The model under review builds one solid part; all positions refer to its coordinate system, in mm. Face numbers are marked on the shaded views. A direction names the side the tool comes from. Round coordinates to 2 decimals unless told otherwise and drop trailing zeros. Order: outer loops, then holes, each group sorted by start corner. A loop starts at its lowest first (then second) coordinate and runs counter-clockwise, first axis right, second up. Notation, with made-up numbers: (11, 0.25) -> (65, 0.25) arc R9 ccw to (65, 15.25) -> close; hole circle Ø8 at (-2.75, 13). An arc over 180 degrees is marked (long way). Use a Markdown table: item, result. Add a question column.
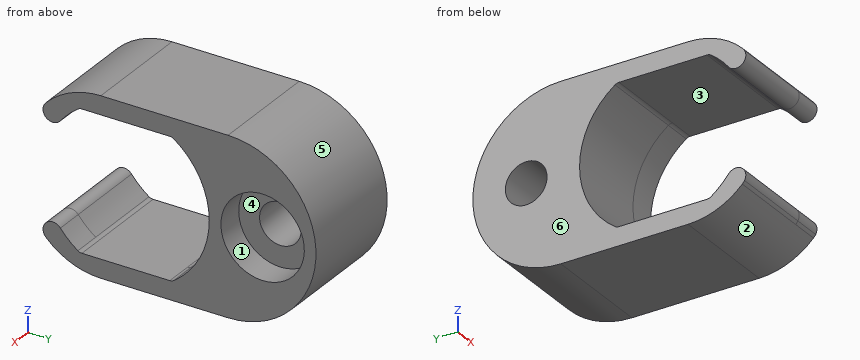
Autodesk Inventor part; units mm, degrees
ref_plane "Work Plane1" through (124.425, 27.025, -10.85) normal (1, 0, 0) x (0, 1, 0)
ref_plane "YZ Plane" through (0, 0, 0) normal (1, 0, 0) x (0, 1, 0)
ref_plane "XZ Plane" through (0, 0, 0) normal (0, 1, 0) x (-1, 0, 0)
sketch "Sketch1" plane through (0, 0, 0) normal (1, 0, 0) x (0, 1, 0)
  line L0 (14.875, -0.7) -> (14.875, 0.8967)
  line L1 (27.025, -0.7) -> (14.875, -0.7)
  line L2 (27.025, -10.85) -> (27.025, -0.7)
  line L3 (15.75, -10.85) -> (27.025, -10.85)
  line L4 (34.625, -12.1) -> (15.75, -12.1)
  line L5 (34.625, -3.2) -> (34.625, -12.1)
  line L6 (15.7197, 0.55) -> (30.875, 0.55)
  arc A0 (17.7877, -0.775) -> (17.5002, -0.8659) centre (17.7877, -1.275) ccw
  arc A1 (17.5002, -0.8659) -> (17.5002, -10.6841) centre (20.95, -5.775) ccw
  arc A2 (17.5002, -10.6841) -> (17.7877, -10.775) centre (17.7877, -10.275) ccw
  line L7 (17.7877, -10.775) -> (24.1123, -10.775)
  arc A3 (24.1123, -10.775) -> (24.3998, -10.6841) centre (24.1123, -10.275) ccw
  arc A4 (24.3998, -10.6841) -> (24.3998, -0.8659) centre (20.95, -5.775) ccw
  arc A5 (24.3998, -0.8659) -> (24.1123, -0.775) centre (24.1123, -1.275) ccw
  line L8 (24.1123, -0.775) -> (17.7877, -0.775)
  line L9 (26.95, -5.775) -> (26.95, -9.775)
  arc A6 (24.3998, -10.6841) -> (26.95, -5.775) centre (20.95, -5.775) ccw
  arc A7 (24.1123, -10.775) -> (24.3998, -10.6841) centre (24.1123, -10.275) ccw
  line L10 (25.95, -10.775) -> (24.1123, -10.775)
  arc A8 (25.95, -10.775) -> (26.95, -9.775) centre (25.95, -9.775) ccw
  line L11 (24.1123, -0.775) -> (25.95, -0.775)
  arc A9 (24.3998, -0.8659) -> (24.1123, -0.775) centre (24.1123, -1.275) ccw
  arc A10 (26.95, -5.775) -> (24.3998, -0.8659) centre (20.95, -5.775) ccw
  line L12 (26.95, -1.775) -> (26.95, -5.775)
  arc A11 (26.95, -1.775) -> (25.95, -0.775) centre (25.95, -1.775) ccw
  line L13 (14.95, -5.775) -> (14.95, -1.775)
  arc A12 (17.5002, -0.8659) -> (14.95, -5.775) centre (20.95, -5.775) ccw
  arc A13 (17.7877, -0.775) -> (17.5002, -0.8659) centre (17.7877, -1.275) ccw
  line L14 (15.95, -0.775) -> (17.7877, -0.775)
  arc A14 (15.95, -0.775) -> (14.95, -1.775) centre (15.95, -1.775) ccw
  line L15 (17.7877, -10.775) -> (15.95, -10.775)
  arc A15 (17.5002, -10.6841) -> (17.7877, -10.775) centre (17.7877, -10.275) ccw
  arc A16 (14.95, -5.775) -> (17.5002, -10.6841) centre (20.95, -5.775) ccw
  line L16 (14.95, -9.775) -> (14.95, -5.775)
  arc A17 (14.95, -9.775) -> (15.95, -10.775) centre (15.95, -9.775) ccw
  line L17 (26.95, -10.85) -> (14.95, -10.85)
  line L18 (14.95, -10.85) -> (14.95, -12.1)
  line L19 (14.95, -12.1) -> (26.95, -12.1)
  line L20 (26.95, -12.1) -> (26.95, -10.85)
  line L21 (20.95, -5.775) -> (14.95, -5.775)
  arc A18 (15.2429, -10.4821) -> (19.1488, -12.1) centre (19.1488, -6.5762) ccw
  arc A19 (15.8269, -8.8981) -> (14.95, -9.775) centre (15.8269, -9.775) ccw
  line L22 (14.95, -9.775) -> (15.8269, -8.8981) construction
  line L23 (14.95, -9.775) -> (16.1901, -9.775) construction
  line L24 (26.95, -0.7) -> (14.95, -0.7)
  line L25 (14.95, -0.7) -> (14.95, 0.55)
  line L26 (14.95, 0.55) -> (26.95, 0.55)
  line L27 (26.95, 0.55) -> (26.95, -0.7)
  arc A20 (19.1488, 0.55) -> (15.2429, -1.0679) centre (19.1488, -4.9738) ccw
  arc A21 (14.95, -1.775) -> (15.8269, -2.6519) centre (15.8269, -1.775) ccw
  line L28 (26.95, -12.1) -> (26.95, 0.55)
  line L29 (26.95, 0.55) -> (34.625, 0.55)
  line L30 (34.625, 0.55) -> (34.625, -12.1)
  line L31 (34.625, -12.1) -> (26.95, -12.1)
  line L32 (26.95, -5.775) -> (34.625, -5.775)
  circle A22 centre (30.7875, -5.775) radius 1.5
  circle A23 centre (30.7875, -5.775) radius 3
  arc A24 (28.3, -12.1) -> (34.625, -5.775) centre (28.3, -5.775) ccw
  arc A25 (34.625, -5.775) -> (28.3, 0.55) centre (28.3, -5.775) ccw
  line L33 (15.75, -12.1) -> (15.75, -10.85)
  arc A26 (34.625, -3.2) -> (30.875, 0.55) centre (30.875, -3.2) ccw
  arc A27 (14.8505, 1.3251) -> (15.7197, 0.55) centre (15.7197, 1.425) ccw
  arc A28 (14.875, 0.8967) -> (14.8505, 1.3251) centre (11.125, 0.8967) ccw
  circle A29 centre (30.7875, -5.775) radius 1.4375
  point P0 (0, 0)
  point P1 (15.8269, -8.8981)
  point P2 (19.1488, -12.1)
  point P3 (28.3, -12.1)
  point P4 (28.3, 0.55)
  point P5 (19.1488, 0.55)
  point P6 (15.2429, -1.0679)
  point P7 (15.8269, -2.6519)
  point P8 (15.75, -10.9306)
  point P9 (27.025, -5.775)
  point P10 (15.6492, -0.7)
  dimension "d0" = 1.25
  dimension "d1" = 45
  dimension "d2" = 3
  dimension "d3" = 6
ref_plane "Work Plane1" through (124.425, 27.025, -10.85) normal (1, 0, 0) x (0, 1, 0)
extrude "Extrusion1" add sketch "Sketch1" along normal blind 6 from surface at 124.425 contours A20 L6 L27 L1 | L1 L28 A11 L11 L8 L14 A14 A20 | L27 L6 A25 L32 A23 L2 L1 | L1 L2 L32 L12 L28 | A14 L14 A0 A1 A21 | L12 A4 A5 L11 A11 | L32 A23 A24 L4 L20 L3 L2 | L2 L3 L28 L9 L32 | L9 A8 L10 A3 A4 | A23 L32 A22 | L32 A22 A23 | L28 L3 L17 A18 A17 L15 L7 L10 A8 | A1 A2 L15 A17 A19 | L20 L4 A18 L33 L3 | L33 A18 L17
fillet "Fillet1" radius 0.7 2 edges at (127.425, 15.8269, -2.6519) (127.425, 15.8269, -8.8981)
sketch "Sketch2" plane through (130.425, 19.1488, -12.1) normal (1, 0, 0) x (0, 0, -1)
  arc A0 (-2.6078, -2.9087) -> (-1.8221, -4.0632) centre (-2.1741, -3.4581) ccw
  line L0 (0, 9.1512) -> (0, 0)
  line L1 (-12.65, 0) -> (-12.65, 9.1512)
  arc A1 (-11.0321, -3.9059) -> (-10.8279, -4.0632) centre (-10.325, -3.1988) ccw
  arc A2 (-11.2341, -1.6486) -> (-10.0422, -2.9087) centre (-6.325, 1.8012) ccw
  arc A3 (-11.325, -1.3611) -> (-11.2341, -1.6486) centre (-10.825, -1.3611) ccw
  arc A4 (-2.6078, -2.9087) -> (-1.4159, -1.6486) centre (-6.325, 1.8012) ccw
  circle A5 centre (-6.325, 11.6387) radius 1.5
  circle A6 centre (-6.325, 11.6387) radius 3
  arc A7 (-1.8221, -4.0632) -> (-1.6179, -3.9059) centre (-2.325, -3.1988) ccw
  arc A8 (-1.6179, -3.9059) -> (0, 0) centre (-5.5238, 0) ccw
  arc A9 (0, 9.1512) -> (-12.65, 9.1512) centre (-6.325, 9.1512) ccw
  arc A10 (-12.65, 0) -> (-11.0321, -3.9059) centre (-7.1262, 0) ccw
  arc A11 (-10.8279, -4.0632) -> (-10.0422, -2.9087) centre (-10.4759, -3.4581) ccw
  line L2 (-11.325, 4.9634) -> (-11.325, -1.3611)
  arc A12 (-11.2341, 5.2509) -> (-11.325, 4.9634) centre (-10.825, 4.9634) ccw
  arc A13 (-1.4159, 5.2509) -> (-11.2341, 5.2509) centre (-6.325, 1.8012) ccw
  arc A14 (-1.325, 4.9634) -> (-1.4159, 5.2509) centre (-1.825, 4.9634) ccw
  line L3 (-1.325, -1.3611) -> (-1.325, 4.9634)
  arc A15 (-1.4159, -1.6486) -> (-1.325, -1.3611) centre (-1.825, -1.3611) ccw
  point P0 (-12.1, -19.1488)
  dimension "d7" = 6
extrude "Extrusion2" add sketch "Sketch2" along normal blind 2 contours A4 A15 L3 A14 A13 A12 L2 A3 A2 A11 A1 A10 L1 A9 L0 A8 A7 A0
properties part number "X Stage Motor Clamp V5"
Q1. Mouldability with a two-part tool opening along Y and no side actions: class the marked faces 4, 5 and 6 as pulls with the +Y half, pulls with the -Y half, needs draft (parallel to the pull), parting line crosses it, or undercut.
Q2. Wall thickness on line 1 (Z direction, x = 132.25, y = 21.25) (3 decimals); line 2 (Z direction, x = 129.75, y = 17); line 3 (Y direction, x = 130.75, z = -10): over which ranges is each line inside the solid? List them lowest first. Write a range as [from, to].
Q3. Add section B-B (z = -6.5). Write out the cut boundary in (x, y) (3 decimals).
Q4. Add section A-A (y = 23.5). Write out the cut boundary in (x, z) (3 decimals).
Q5. Insertion check: pin 1 (1.8 mm diameter, centred on y = 30.5, z = -6, fed in from +X); pin 2 (1 mm diameter, centred on x = 130, z = -5.5, fed in from -Y); pin 3 (3.5 mm diameter, centred on y = 30.79, z = -5.78, fed in from +X) (3 decimals); pin 4 (1.5 mm diameter, centred on x = 125.5, y = 31.5, fed in from +Z). Each pin has a flat end and moves straight along its axis. Give the tip position at first contact, or say it passes through.
Q6. Add section D-D (y = 30.25). Write out the cut boundary in (x, z) (3 decimals).
Q7. Add section C-C (z = -8.5). Write out the cut boundary in (x, y) (3 decimals), then the cut area to 3 significant figures.
Q8. Machinability: for the marked faces 1, 2 and 3, which of the approach directions +Z, -Z, +X, -X, +Y, -Y give a long, thin tool a straight path to every point of the face, cutting with its end or side? Answer none if there is none.
Report:
| question | item | result |
|---|---|---|
| 1 | face 4 | undercut |
| 1 | face 5 | pulls with the +Y half |
| 1 | face 6 | needs draft |
| 2 | line 1 | z = [-12.1, -10.775], [-0.775, 0.55] |
| 2 | line 2 | z = [-11.66, -10.29], [-1.26, 0.11] |
| 2 | line 3 | y = [14.99, 16.69], [25.21, 33.01] |
| 3 | outline | (124.425, 26.906) -> (132.425, 26.906) -> (132.425, 27.876) -> (130.425, 27.876) -> (130.425, 29.474) -> (124.425, 29.474) -> close; (124.425, 32.101) -> (130.425, 32.101) -> (130.425, 33.699) -> (132.425, 33.699) -> (132.425, 34.583) -> (124.425, 34.583) -> close |
| 4 | outline | (124.425, -12.1) -> (132.425, -12.1) -> (132.425, -10.775) -> (124.425, -10.775) -> close; (124.425, -0.775) -> (132.425, -0.775) -> (132.425, 0.55) -> (124.425, 0.55) -> close |
| 5 | pin 1 | passes through |
| 5 | pin 2 | stops at y = 26.9 |
| 5 | pin 3 | stops at x = 130.425 |
| 5 | pin 4 | stops at z = 0.06 |
| 6 | outline | (124.425, -11.792) -> (132.425, -11.792) -> (132.425, -8.726) -> (130.425, -8.726) -> (130.425, -7.175) -> (124.425, -7.175) -> close; (124.425, -4.375) -> (130.425, -4.375) -> (130.425, -2.824) -> (132.425, -2.824) -> (132.425, 0.242) -> (124.425, 0.242) -> close |
| 7 | outline | (124.425, 26.296) -> (132.425, 26.295) -> (132.425, 29.533) -> (130.425, 29.533) -> (130.425, 32.042) -> (132.425, 32.042) -> (132.425, 34.008) -> (124.425, 34.008) -> close |
| 7 | area | 56.7 mm² |
| 8 | face 1 | +X |
| 8 | face 2 | -Z, +X, -X, -Y |
| 8 | face 3 | +X, -X |
